Here's how the part is built. I have some questions about the finished solid (model axes, mm). Coordinates: 2 decimals unless noted, no trailing zeros. Write each loop counter-clockwise with the first axis right and the second up, starting at its lowest first coordinate (ties: lowest second). Pieces come first, ordered by that corner, then holes.
Item 1: Please list where these lines run through material, in increasing order: line 1 (X direction, y = 1, z = -0.2); line 2 (X direction, y = 1.25, z = -0.7).
Item 2: I want a section at A-A (y = 0). Please give me the cut outline in (x, z), and give its area (3 significant figures).
Item 3: I want a section at B-B (z = -1.15). Please give me the cut outline in (x, y).
Item 4: If we mould it in two halves opening along X, with no side actions, what happens to faces 1 (the face through (31.37, 0.09, -0.8)), 2 (the face through (38.1, 0, -1)), 3 (the face through (-1, 12.7, -1))? For each: pulls with the +X half, pulls with the -X half, needs draft (parallel to the pull), parting line crosses it, or undercut.
from build123d import *

# Parameters (mm, degrees)
SKETCH1_W           = 76.2
SKETCH1_H           = 25.4
BOSS_EXTRUDE1_DEPTH = 1.6256
SKETCH2_R           = 2.159
CUT_EXTRUDE1_DEPTH  = 41.19381265


with BuildPart() as part:
    # Sketch1 → Boss-Extrude1 (new body)
    with BuildSketch(Plane.XY):
        Rectangle(SKETCH1_W, SKETCH1_H)
    extrude(amount=-BOSS_EXTRUDE1_DEPTH)

    # Sketch2 → Cut-Extrude1 (cut, through all)
    with BuildSketch(Plane.XY):
        with Locations((33.528, 0)):
            Circle(SKETCH2_R)
        with Locations(Location((-33.528, 0, 0), (0, 0, 180))):
            Circle(SKETCH2_R)
    extrude(amount=-CUT_EXTRUDE1_DEPTH, mode=Mode.SUBTRACT)


solid = part.part
Answer:
1. line 1: x = -38.1 to -35.44, -31.61 to 31.61, 35.44 to 38.1
1. line 2: x = -38.1 to -35.29, -31.77 to 31.77, 35.29 to 38.1
2. outline: (-38.1, -1.63) - (-35.69, -1.63) - (-35.69, 0) - (-38.1, 0) - close; (-31.37, -1.63) - (31.37, -1.63) - (31.37, 0) - (-31.37, 0) - close; (35.69, -1.63) - (38.1, -1.63) - (38.1, 0) - (35.69, 0) - close
2. area: 110 mm2
3. outline: (-38.1, -12.7) - (38.1, -12.7) - (38.1, 12.7) - (-38.1, 12.7) - close; hole circle Ø4.32 at (-33.53, 0); hole circle Ø4.32 at (33.53, 0)
4. face 1: undercut
4. face 2: pulls with the +X half
4. face 3: needs draft
